Can you work these out from the model? Positions are in its coordinate system, mm. Give positions to 0.01 mm unless a question says otherwise; leave off trailing zeros. Loops run counter-clockwise (first coordinate to the right, second up) from the corner with the lowest first, then second, coordinate; pieces in that order, holes last. Notation, with made-up numbers: (86, 49.5) - (105, 49.5) arc R15 ccw to (105, 73.5) - close; hole circle Ø2 at (-23.75, 40). An arc over 180 degrees is marked (long way). Use a Markdown table: item, result. Add a question column.
```python
from build123d import *

# Parameters (mm, degrees)
BOSS_EXTRUDE1_DEPTH = 2.032
SKETCH2_R           = 1.905
CUT_EXTRUDE1_DEPTH  = 21.617854496


with BuildPart() as part:
    # Sketch1 → Boss-Extrude1 (new body)
    with BuildSketch(Plane(origin=(0, 0, 0), x_dir=(1, 0, 0), z_dir=(0, 1, 0))):
        with BuildLine():
            Line((0, 0), (15.24, 0))
            ThreePointArc((15.24, 0), (19.05, -3.81), (15.24, -7.62))
            Line((15.24, -7.62), (0, -7.62))
            Line((0, -7.62), (0, 0))
        make_face()
    extrude(amount=BOSS_EXTRUDE1_DEPTH)

    # Sketch2 → Cut-Extrude1 (cut, through all)
    with BuildSketch(Plane(origin=(0, 2.032, 0), x_dir=(1, 0, 0), z_dir=(0, 1, 0))):
        with Locations(Location((15.24, -3.81, 0), (0, 0, 270))):
            Circle(SKETCH2_R)
    extrude(amount=-CUT_EXTRUDE1_DEPTH, mode=Mode.SUBTRACT)


solid = part.part
```
1. Please list where these lines run through material, in increasing order: line 1 along X through (y, z) = (0.8, 3.81) (3 decimals); line 2 along X through (y, z) = (0.85, 5.25); line 3 along Z through (x, y) = (16.75, 0.35). Write a range as [from, to].
2. Suppose I cut it at D-D (z = 7). List the corners of the cut face in (x, y) for me, and give its area (3 significant figures).
3. Suppose I cut it at C-C (x = 16.5). List the corners of the cut face in (y, z) for me.
4. Suppose I cut it at B-B (y = 1.6). List the corners of the cut face in (x, z) for me (3 decimals).
5. Suppose I cut it at A-A (z = 3.81). List the corners of the cut face in (x, y) for me (3 decimals), and give its area (3 significant figures).
6. If we mould it in two halves opening along Z, with no side actions, what happens to faces 1 (the face through (13.55, 1.03, 4.69)), 2 (the face through (10, 0, 4)), 3 (the face through (19.05, 1, 3.73)), 4 (the face through (8, 1, 0))? For each: released by +Z, released by -Z, zero draft, split by the parting line, or undercut.
7. Will this pin go through, and if not, where does the flat tip stop? P1, Ø3, axis at x = 15.24, z = 3.81, coming from the -Y side.
Results below:
| question | item | result |
|---|---|---|
| 1 | line 1 | [0, 13.335], [17.145, 19.05] |
| 1 | line 2 | [0, 13.99], [16.49, 18.77] |
| 1 | line 3 | [0.31, 2.65], [4.97, 7.31] |
| 2 | outline | (0, 0) - (17.32, 0) - (17.32, 2.03) - (0, 2.03) - close |
| 2 | area | 35.2 mm² |
| 3 | outline | (0, 0.21) - (2.03, 0.21) - (2.03, 2.38) - (0, 2.38) - close; (0, 5.24) - (2.03, 5.24) - (2.03, 7.41) - (0, 7.41) - close |
| 4 | outline | (0, 0) - (15.24, 0) arc R3.81 ccw to (15.24, 7.62) - (0, 7.62) - close; hole circle Ø3.81 at (15.24, 3.81) |
| 5 | outline | (0, 0) - (13.335, 0) - (13.335, 2.032) - (0, 2.032) - close; (17.145, 0) - (19.05, 0) - (19.05, 2.032) - (17.145, 2.032) - close |
| 5 | area | 31.0 mm² |
| 6 | face 1 | undercut |
| 6 | face 2 | zero draft |
| 6 | face 3 | split by the parting line |
| 6 | face 4 | released by -Z |
| 7 | P1 | through |
